from build123d import *

# Parameters (mm, degrees)
SKETCH_1_W        = 6
SKETCH_1_H        = 15
EXTRUDE_3_DEPTH   = 15
SKETCH_1_7_W      = 6
SKETCH_1_7_H      = 15
EXTRUDE_3_2_DEPTH = 15
EXTRUDE_4_DEPTH   = 15
SKETCH_1_11_W     = 18
SKETCH_1_11_H     = 18
SKETCH_1_11_W_2   = 6
SKETCH_1_11_H_2   = 15
SKETCH_1_11_W_3   = 15
SKETCH_1_11_H_3   = 6
SKETCH_1_11_W_4   = 7
EXTRUDE_5_DEPTH   = 5
SKETCH_1_13_W     = 3
SKETCH_1_13_H     = 40
EXTRUDE_10_DEPTH  = 20
SKETCH_3_W        = 14.869090603
SKETCH_3_H        = 6
EXTRUDE_15_DEPTH  = 15


with BuildPart() as part:
    # Sketch 1 → Extrude 3 (new body)
    with BuildSketch(Plane.XY):
        with Locations((-25.796959303, 23.532605762)):
            Rectangle(SKETCH_1_W, SKETCH_1_H)
    extrude(amount=EXTRUDE_3_DEPTH)



with BuildPart() as body_2:
    # Sketch 1_7 → Extrude 3 2 (new body)
    with BuildSketch(Plane.XY):
        with Locations((-74.796959303, 23.532605762)):
            Rectangle(SKETCH_1_7_W, SKETCH_1_7_H)
    extrude(amount=EXTRUDE_3_2_DEPTH)


with BuildPart() as body_3:
    # Sketch 1_8 → Extrude 4 (new body)
    with BuildSketch(Plane.XY):
        Polygon((-71.796959303, 49.032605762), (-68.796959303, 49.032605762), (-50.796959303, 49.032605762), (-28.796959303, 49.032605762), (-28.796959303, 52.032605762), (-35.796959303, 52.032605762), (-50.796959303, 52.032605762), (-71.796959303, 52.032605762), align=None)
    extrude(amount=EXTRUDE_4_DEPTH)


with BuildPart() as part_1:
    add(part.part)

    add(body_2.part)  # Extrude 5 merges body 2

    add(body_3.part)  # Extrude 5 merges body 3
    # Sketch 1_11 → Extrude 5 (add)
    with BuildSketch(Plane.XY):
        Polygon((-68.796959303, 9.032605762), (-50.796959303, 9.032605762), (-35.796959303, 9.032605762), (-35.796959303, 3.032605762), (-28.796959303, 3.032605762), (-28.796959303, 9.032605762), (-22.796959303, 9.032605762), (-22.796959303, 16.032605762), (-28.796959303, 16.032605762), (-28.796959303, 31.032605762), (-28.796959303, 49.032605762), (-50.796959303, 49.032605762), (-50.796959303, 31.032605762), (-68.796959303, 31.032605762), align=None)
        with Locations((-59.796959303, 40.032605762)):
            Rectangle(SKETCH_1_11_W, SKETCH_1_11_H)
        with Locations((-25.796959303, 23.532605762)):
            Rectangle(SKETCH_1_11_W_2, SKETCH_1_11_H_2)
        with Locations((-74.796959303, 23.532605762)):
            Rectangle(SKETCH_1_11_W_2, SKETCH_1_11_H_2)
        Polygon((-71.796959303, 9.032605762), (-68.796959303, 9.032605762), (-68.796959303, 31.032605762), (-68.796959303, 49.032605762), (-71.796959303, 49.032605762), (-71.796959303, 31.032605762), (-71.796959303, 16.032605762), align=None)
        Polygon((-71.796959303, 49.032605762), (-68.796959303, 49.032605762), (-50.796959303, 49.032605762), (-28.796959303, 49.032605762), (-28.796959303, 52.032605762), (-35.796959303, 52.032605762), (-50.796959303, 52.032605762), (-71.796959303, 52.032605762), align=None)
        with Locations((-43.296959303, 55.032605762)):
            Rectangle(SKETCH_1_11_W_3, SKETCH_1_11_H_3)
        with Locations((-32.296959303, 55.032605762)):
            Rectangle(SKETCH_1_11_W_4, SKETCH_1_11_H_3)
        with Locations((-43.296959303, 6.032605762)):
            Rectangle(SKETCH_1_11_W_3, SKETCH_1_11_H_3)
    extrude(amount=-EXTRUDE_5_DEPTH)

    # Sketch 1_13 → Extrude 10 (add)
    with BuildSketch(Plane.XY):
        with Locations((-70.296959303, 29.032605762)):
            Rectangle(SKETCH_1_13_W, SKETCH_1_13_H)
    extrude(amount=-EXTRUDE_10_DEPTH)

    # Sketch 3 → Extrude 15 (add)
    with BuildSketch(Plane(origin=(0, 0, -5), x_dir=(-1, 0, 0), z_dir=(0, 0, -1))):
        with Locations((43.362414001, 55.032605762)):
            Rectangle(SKETCH_3_W, SKETCH_3_H)
        with Locations((43.362414001, 6.032605762)):
            Rectangle(SKETCH_3_W, SKETCH_3_H)
    extrude(amount=EXTRUDE_15_DEPTH)


solid = part_1.part
Design review of the part built by this model. Coordinates are the model's own, in mm. A direction names the side the tool comes from. Give positions to 0.01 mm unless a question says otherwise; leave off trailing zeros. Write each loop counter-clockwise with the first axis right and the second up, starting at its lowest first coordinate (ties: lowest second). Pieces come first, ordered by that corner, then holes. Notation, with made-up numbers: M 45,71.25 L 98,71.25 A13 cw 98,83.25 Z; hole C 84,73.25 d10. An arc over 180 degrees is marked long. Return JSON: item names as keys, results as strings. Group by question number.
Item 1: Take a section at D-D (z = 11). Give the boundary of the cut face in (x, y), plus the area to 3 significant figures.
Item 2: Take a section at A-A (z = -10). Give the boundary of the cut face in (x, y), plus the area to 3 significant figures.
Item 3: Wall thickness on line 1 along Y through (x, z) = (-43, -8.5); line 2 along Y through (x, z) = (-55, -3); line 3 along Z through (x, y) = (-33.5, 17): over which ranges is each line inside the solid? List them lowest first.
Item 4: Tool access review of faces 1 (the flat face through (-26, 31.033, 5)), 2 (the flat face through (-75, 31.033, 5)), 3 (the flat face through (-43, 52.033, -12)), 4 (the flat face through (-28.797, 6, -2)): name each direction out of +Z, -Z, +X, -X, +Y, -Y from which nothing blocks a thin tool from reaching the whole face with its end or side.
Item 5: Clearance check with flat-ended pins moving along their axes: pin 1 Ø3 at (x, z) = (-57.5, 0.5) entering from +Y; pin 2 Ø1.8 at (y, z) = (55, -14.5) entering from +X; pin 3 Ø7.5 at (y, z) = (36, -11) entering from +X. State where each tip first meets the part, or that it passes through.
Item 6: The part is to be moulded in two halves that separate along Y. For faces 5 (the flat face through (-48, 31, -5)), 6 (the flat face through (-70, 29, -20)), 7 (the flat face through (-63.7, 9.033, -4.8)), say which applies: pulls with the +Y half, pulls with the -Y half, needs draft (parallel to the pull), parting line crosses it, or undercut.
Item 7: Take a section at B-B (y = 23.5). Give the boundary of the cut face in (x, z), plus the area to 3 significant figures.
Item 8: Take a section at C-C (x = -49). Give the boundary of the cut face in (y, z).
Return value:
{
 "1": {"outline": "M -77.8,16.03 L -71.8,16.03 L -71.8,31.03 L -77.8,31.03 Z; M -71.8,49.03 L -28.8,49.03 L -28.8,52.03 L -71.8,52.03 Z; M -28.8,16.03 L -22.8,16.03 L -22.8,31.03 L -28.8,31.03 Z", "area": "309 mm2"},
 "2": {"outline": "M -71.8,9.03 L -68.8,9.03 L -68.8,49.03 L -71.8,49.03 Z; M -50.8,3.03 L -35.93,3.03 L -35.93,9.03 L -50.8,9.03 Z; M -50.8,52.03 L -35.93,52.03 L -35.93,58.03 L -50.8,58.03 Z", "area": "298 mm2"},
 "3": {"line 1": "y = 3.03 to 9.03, 52.03 to 58.03", "line 2": "y = 9.03 to 52.03", "line 3": "z = -5 to 0"},
 "4": {"face 1": "+Z, -Z, +X, +Y", "face 2": "+Z, -Z, -X, +Y", "face 3": "-Z, +X, -X", "face 4": "+Z, -Z, +X, -Y"},
 "5": {"pin 1": "stops at y = 52.03", "pin 2": "stops at x = -35.93", "pin 3": "stops at x = -68.8"},
 "6": {"face 5": "undercut", "face 6": "needs draft", "face 7": "pulls with the -Y half"},
 "7": {"outline": "M -77.8,-5 L -71.8,-5 L -71.8,-20 L -68.8,-20 L -68.8,-5 L -22.8,-5 L -22.8,15 L -28.8,15 L -28.8,0 L -71.8,0 L -71.8,15 L -77.8,15 Z", "area": "500 mm2"},
 "8": {"outline": "M 3.03,-20 L 9.03,-20 L 9.03,-5 L 52.03,-5 L 52.03,-20 L 58.03,-20 L 58.03,0 L 52.03,0 L 52.03,15 L 49.03,15 L 49.03,0 L 3.03,0 Z"}
}
